```python
from build123d import *

# Parameters (mm, degrees)
SKETCH1_R            = 12.827
BOSS_EXTRUDE1_DEPTH  = 38.1
SKETCH2_W            = 25.654
SKETCH2_H            = 25.4
BOSS_EXTRUDE2_DEPTH  = 3.302
SKETCH8_W            = 63.5
SKETCH8_H            = 38.1
BOSS_EXTRUDE6_DEPTH  = 8.89
SKETCH10_W           = 38.1
SKETCH10_H           = 46.99
BOSS_EXTRUDE7_DEPTH  = 1.016
SKETCH11_W           = 38.1
SKETCH11_H           = 46.99
BOSS_EXTRUDE8_DEPTH  = 1.016
SKETCH13_W           = 25.4
SKETCH13_H           = 38.1
BOSS_EXTRUDE9_DEPTH  = 1.524
SKETCH14_W           = 25.4
SKETCH14_H           = 38.1
BOSS_EXTRUDE10_DEPTH = 1.524


with BuildPart() as part:
    # Sketch1 → Boss-Extrude1 (new body)
    with BuildSketch(Plane.XY):
        with Locations(Location((0, -30.101764051, 0), (0, 0, 180))):
            Circle(SKETCH1_R)
    extrude(amount=BOSS_EXTRUDE1_DEPTH)

    # Sketch2 → Boss-Extrude2 (add)
    with BuildSketch(Plane.XY):
        with Locations((0, -17.401764051)):
            Rectangle(SKETCH2_W, SKETCH2_H)
    extrude(amount=BOSS_EXTRUDE2_DEPTH)

    # Sketch8 → Boss-Extrude6 (add)
    with BuildSketch(Plane(origin=(0, -4.701764051, 0), x_dir=(1, 0, 0), z_dir=(0, 1, 0))):
        with Locations((0, -19.05)):
            Rectangle(SKETCH8_W, SKETCH8_H)
    extrude(amount=BOSS_EXTRUDE6_DEPTH)

    # Sketch10 → Boss-Extrude7 (add)
    with BuildSketch(Plane(origin=(31.75, 0, 0), x_dir=(0, 0, -1), z_dir=(1, 0, 0))):
        with Locations((-19.05, 18.793235949)):
            Rectangle(SKETCH10_W, SKETCH10_H)
    extrude(amount=BOSS_EXTRUDE7_DEPTH)

    # Sketch11 → Boss-Extrude8 (add)
    with BuildSketch(Plane.ZY.offset(31.75)):
        with Locations((19.05, 18.793235949)):
            Rectangle(SKETCH11_W, SKETCH11_H)
    extrude(amount=BOSS_EXTRUDE8_DEPTH)

    # Sketch13 → Boss-Extrude9 (add)
    with BuildSketch(Plane(origin=(0, 42.288235949, 0), x_dir=(1, 0, 0), z_dir=(0, 1, 0))):
        with Locations((20.066, -19.05)):
            Rectangle(SKETCH13_W, SKETCH13_H)
    extrude(amount=BOSS_EXTRUDE9_DEPTH)

    # Sketch14 → Boss-Extrude10 (add)
    with BuildSketch(Plane(origin=(0, 42.288235949, 0), x_dir=(1, 0, 0), z_dir=(0, 1, 0))):
        with Locations((-20.066, -19.05)):
            Rectangle(SKETCH14_W, SKETCH14_H)
    extrude(amount=BOSS_EXTRUDE10_DEPTH)


solid = part.part
```
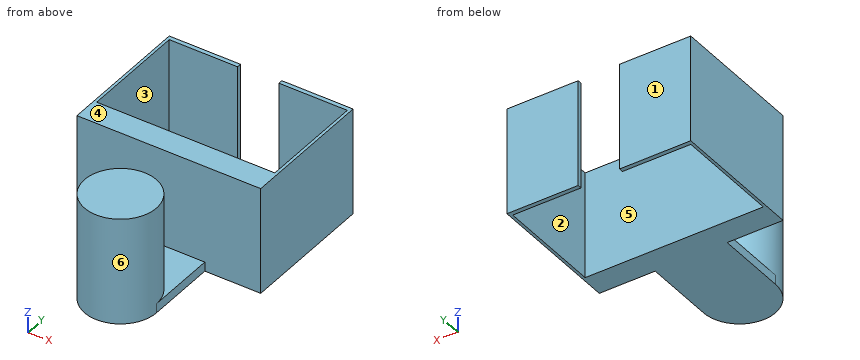
Geometry check sheet. Reference: the model listing, model coordinates, mm. Face numbers are marked on the shaded views. A direction names the side the tool comes from. Round coordinates to 2 decimals unless told otherwise and drop trailing zeros. Order: outer loops, then holes, each group sorted by start corner. A loop starts at its lowest first (then second) coordinate and runs counter-clockwise, first axis right, second up. Notation, with made-up numbers: (6.5, -2) - (25.5, -2) arc R28 ccw to (25.5, 27) - close; hole circle Ø4 at (-28.5, -39.5). An arc over 180 degrees is marked (long way). Use a Markdown table: item, result. Add a question column.
1) Section check C-C (x = 27). Record the cut outline in (y, z), then the cut area to 3 significant figures.
2) Section check A-A (y = 35.5). Record the cut outline in (x, z), then the cut area to 3 significant figures.
3) Set-up check for the marked faces 1 and 2: record each of +Z, -Z, +X, -X, +Y, -Y from which the full face is reachable in a straight line by a thin tool's end or side.
4) Thickness scan on line 1 along X through (y, z) = (31, 29.5); line 2 along Y through (x, z) = (14.5, 6); line 3 along Y through (x, z) = (9, 7). Record the ranges inside material, lowest first.
5) Gauge pin test, flat ends, axial feed: P1, Ø2.5, axis at y = -19, z = 1, coming from the -X side; P2, Ø7.5, axis at x = -6.5, y = -14, coming from the +Z side; P3, Ø11.5, axis at x = 8.5, z = 13.5, coming from the -Y side. Record the tip position at first contact, or that the pin passes through.
6) Section check B-B (z = 14.5). Record the cut outline in (x, y).
7) Mould release check, pull along X, two halves, no side actions. Record for the marked faces 3, 4, 5 and 6: released by +X, released by -X, zero draft, split by the parting line, or undercut.
8) Section check D-D (x = 0). Record the cut outline in (y, z), then the cut area to 3 significant figures.
Established:
| question | item | result |
|---|---|---|
| 1 | outline | (-4.7, 0) - (4.19, 0) - (4.19, 38.1) - (-4.7, 38.1) - close; (42.29, 0) - (43.81, 0) - (43.81, 38.1) - (42.29, 38.1) - close |
| 1 | area | 397 mm2 |
| 2 | outline | (-32.77, 0) - (-31.75, 0) - (-31.75, 38.1) - (-32.77, 38.1) - close; (31.75, 0) - (32.77, 0) - (32.77, 38.1) - (31.75, 38.1) - close |
| 2 | area | 77.4 mm2 |
| 3 | face 1 | +Z, -Z, +X, -X, +Y |
| 3 | face 2 | +Z, -Z |
| 4 | line 1 | -32.77 to -31.75, 31.75 to 32.77 |
| 4 | line 2 | -4.7 to 4.19, 42.29 to 43.81 |
| 4 | line 3 | -39.24 to -20.96, -4.7 to 4.19, 42.29 to 43.81 |
| 5 | P1 | x = -12.83 |
| 5 | P2 | z = 3.3 |
| 5 | P3 | y = -42.63 |
| 6 | outline | (-32.77, -4.7) - (32.77, -4.7) - (32.77, 43.81) - (7.37, 43.81) - (7.37, 42.29) - (31.75, 42.29) - (31.75, 4.19) - (-31.75, 4.19) - (-31.75, 42.29) - (-7.37, 42.29) - (-7.37, 43.81) - (-32.77, 43.81) - close; circle Ø25.65 at (0, -30.1) |
| 7 | face 3 | undercut |
| 7 | face 4 | zero draft |
| 7 | face 5 | undercut |
| 7 | face 6 | split by the parting line |
| 8 | outline | (-42.93, 0) - (4.19, 0) - (4.19, 38.1) - (-4.7, 38.1) - (-4.7, 3.3) - (-17.27, 3.3) - (-17.27, 38.1) - (-42.93, 38.1) - close |
| 8 | area | 1,360 mm2 |
